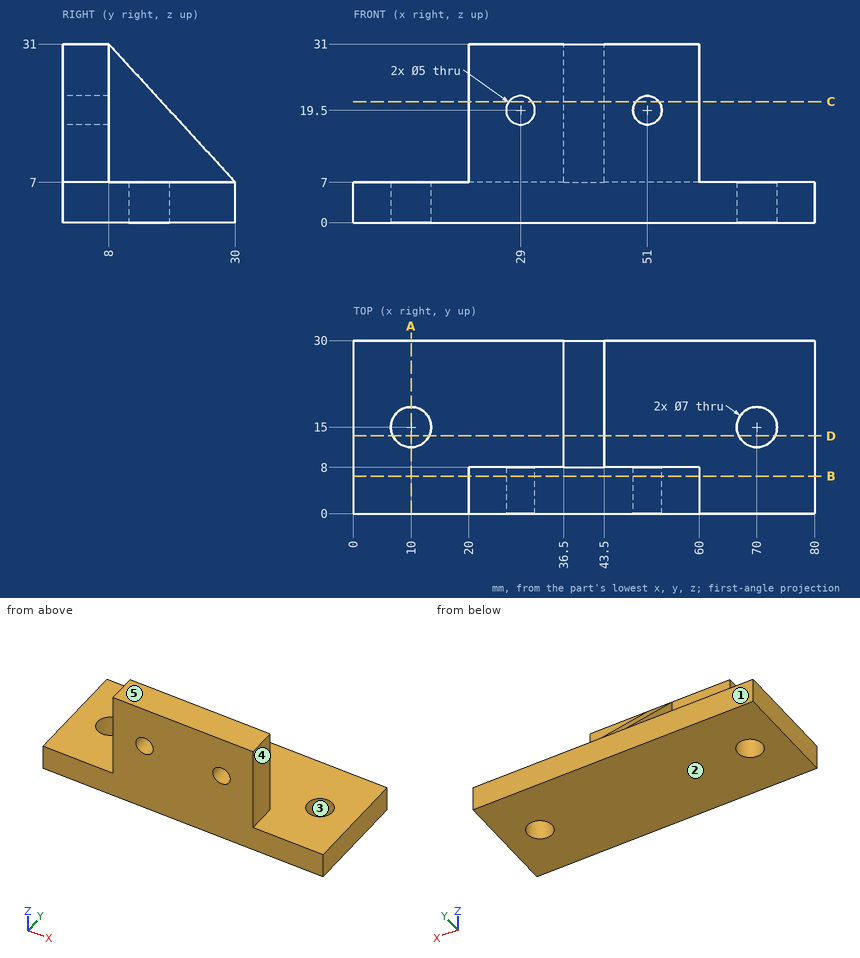
Can you work these out from the drawing? Everything is in mm from the part's minimum corner. A direction names the side the tool comes from. Coordinates: 2 decimals unless noted, no trailing zeros. Loops run counter-clockwise (first coordinate to the right, second up) from the corner with the lowest first, then second, coordinate; pieces in that order, holes last.
1) For pin 1 (15 mm diameter, centred on x = 9.5, y = 11, fed in from +Z); pin 2 (1 mm diameter, centred on x = 29.5, z = 15.5, fed in from +Y); pin 3 (9 mm diameter, centred on y = 5.5, z = 15, fed in from +X), each with a flat end and sliding along its axis, tell me the tip position at first contact or that it passes through.
2) Imagine slicing it at C-C on z = 21. List the corners of the cut face in (x, y) for me, plus the area to 3 significant figures.
3) Imagine slicing it at A-A on x = 10. List the corners of the cut face in (y, z) for me.
4) I need wall thicknesses on probe 1 along X at (y, z) = (15, 1.5); probe 2 along Y at (x, z) = (70, 5.75); probe 3 along X at (y, z) = (2, 19). Which ranges of each line are inside material? Lowest first, please.
5) Thinking about a two-plate mould opening in Y: for the marked faces 1, 2 and 3, which applies, pulls with the +Y half, pulls with the -Y half, needs draft (parallel to the pull), parting line crosses it, or undercut?
6) Which directions (+Z, -Z, +X, -X, +Y, -Y) give clear straight access to the entire face, cutting with the end or side of a thin tool? Please do the marked faces 4 and 5.
7) Imagine slicing it at B-B on y = 6.5. List the corners of the cut face in (x, z) for me, plus the area to 3 significant figures.
8) Imagine slicing it at D-D on y = 13.5. List the corners of the cut face in (x, z) for me.
Completed:
1. pin 1: stops at z = 7
1. pin 2: stops at y = 8
1. pin 3: stops at x = 60
2. outline: (20, 0) - (27, 0) - (27, 8) - (20, 8) - close; (31, 0) - (49, 0) - (49, 8) - (43.5, 8) - (43.5, 17.17) - (36.5, 17.17) - (36.5, 8) - (31, 8) - close; (53, 0) - (60, 0) - (60, 8) - (53, 8) - close
2. area: 320 mm2
3. outline: (0, 0) - (11.5, 0) - (11.5, 7) - (0, 7) - close; (18.5, 0) - (30, 0) - (30, 7) - (18.5, 7) - close
4. probe 1: x = 0 to 6.5, 13.5 to 66.5, 73.5 to 80
4. probe 2: y = 0 to 11.5, 18.5 to 30
4. probe 3: x = 20 to 26.55, 31.45 to 48.55, 53.45 to 60
5. face 1: pulls with the +Y half
5. face 2: needs draft
5. face 3: undercut
6. face 4: +Z, +X, +Y, -Y
6. face 5: +Z, +X, -X, +Y, -Y
7. outline: (0, 0) - (80, 0) - (80, 7) - (60, 7) - (60, 31) - (20, 31) - (20, 7) - (0, 7) - close; hole circle Ø5 at (29, 19.5); hole circle Ø5 at (51, 19.5)
7. area: 1,480 mm2
8. outline: (0, 0) - (6.84, 0) - (6.84, 7) - (0, 7) - close; (13.16, 0) - (66.84, 0) - (66.84, 7) - (43.5, 7) - (43.5, 25) - (36.5, 25) - (36.5, 7) - (13.16, 7) - close; (73.16, 0) - (80, 0) - (80, 7) - (73.16, 7) - close
